from build123d import *

# Parameters (mm, degrees)
SKETCH1_W           = 400
SKETCH1_H           = 70
SKETCH1_R           = 30
SKETCH1_R_2         = 1.5
BOSS_EXTRUDE1_DEPTH = 3


with BuildPart() as part:
    # Sketch1 → Boss-Extrude1 (new body)
    with BuildSketch(Plane(origin=(0, 0, 0), x_dir=(1, 0, 0), z_dir=(0, 1, 0))):
        with Locations((200, 35)):
            Rectangle(SKETCH1_W, SKETCH1_H)
        with Locations(Location((40, 35, 0), (0, 0, 270))):
            Circle(SKETCH1_R, mode=Mode.SUBTRACT)
        with Locations(Location((120, 35, 0), (0, 0, 270))):
            Circle(SKETCH1_R, mode=Mode.SUBTRACT)
        with Locations(Location((200, 35, 0), (0, 0, 270))):
            Circle(SKETCH1_R, mode=Mode.SUBTRACT)
        with Locations(Location((280, 35, 0), (0, 0, 270))):
            Circle(SKETCH1_R, mode=Mode.SUBTRACT)
        with Locations(Location((360, 35, 0), (0, 0, 270))):
            Circle(SKETCH1_R, mode=Mode.SUBTRACT)
        with Locations(Location((15, 60, 0), (0, 0, 270))):
            Circle(SKETCH1_R_2, mode=Mode.SUBTRACT)
        with Locations(Location((65, 60, 0), (0, 0, 270))):
            Circle(SKETCH1_R_2, mode=Mode.SUBTRACT)
        with Locations(Location((65, 10, 0), (0, 0, 270))):
            Circle(SKETCH1_R_2, mode=Mode.SUBTRACT)
        with Locations(Location((15, 10, 0), (0, 0, 270))):
            Circle(SKETCH1_R_2, mode=Mode.SUBTRACT)
        with Locations(Location((95, 60, 0), (0, 0, 270))):
            Circle(SKETCH1_R_2, mode=Mode.SUBTRACT)
        with Locations(Location((145, 60, 0), (0, 0, 270))):
            Circle(SKETCH1_R_2, mode=Mode.SUBTRACT)
        with Locations(Location((145, 10, 0), (0, 0, 270))):
            Circle(SKETCH1_R_2, mode=Mode.SUBTRACT)
        with Locations(Location((95, 10, 0), (0, 0, 270))):
            Circle(SKETCH1_R_2, mode=Mode.SUBTRACT)
        with Locations(Location((175, 60, 0), (0, 0, 270))):
            Circle(SKETCH1_R_2, mode=Mode.SUBTRACT)
        with Locations(Location((225, 60, 0), (0, 0, 270))):
            Circle(SKETCH1_R_2, mode=Mode.SUBTRACT)
        with Locations(Location((225, 10, 0), (0, 0, 270))):
            Circle(SKETCH1_R_2, mode=Mode.SUBTRACT)
        with Locations(Location((175, 10, 0), (0, 0, 270))):
            Circle(SKETCH1_R_2, mode=Mode.SUBTRACT)
        with Locations(Location((255, 60, 0), (0, 0, 270))):
            Circle(SKETCH1_R_2, mode=Mode.SUBTRACT)
        with Locations(Location((305, 60, 0), (0, 0, 270))):
            Circle(SKETCH1_R_2, mode=Mode.SUBTRACT)
        with Locations(Location((305, 10, 0), (0, 0, 270))):
            Circle(SKETCH1_R_2, mode=Mode.SUBTRACT)
        with Locations(Location((255, 10, 0), (0, 0, 270))):
            Circle(SKETCH1_R_2, mode=Mode.SUBTRACT)
        with Locations(Location((335, 60, 0), (0, 0, 270))):
            Circle(SKETCH1_R_2, mode=Mode.SUBTRACT)
        with Locations(Location((385, 60, 0), (0, 0, 270))):
            Circle(SKETCH1_R_2, mode=Mode.SUBTRACT)
        with Locations(Location((385, 10, 0), (0, 0, 270))):
            Circle(SKETCH1_R_2, mode=Mode.SUBTRACT)
        with Locations(Location((335, 10, 0), (0, 0, 270))):
            Circle(SKETCH1_R_2, mode=Mode.SUBTRACT)
    extrude(amount=BOSS_EXTRUDE1_DEPTH)


solid = part.part
The model under review builds one solid part; all positions refer to its coordinate system, in mm. Coordinates: 2 decimals unless noted, no trailing zeros. Loops run counter-clockwise (first coordinate to the right, second up) from the corner with the lowest first, then second, coordinate; pieces in that order, holes last.
(1) Insertion check: P1, Ø2.5, axis at x = 385, z = -60, coming from the +Y side; P2, Ø5, axis at x = 95, z = -10, coming from the +Y side. Each pin has a flat end and moves straight along its axis. Give the tip position at first contact, or say it passes through.
Determined:
P1: passes through
P2: stops at y = 3
(2) Consider section A-A, the plane x = 280. Give the boundary of the cut face in (y, z).
Determined:
outline: (0, -70) - (3, -70) - (3, -65) - (0, -65) - close; (0, -5) - (3, -5) - (3, 0) - (0, 0) - close
(3) Consider section B-B, the plane z = -53. Give the boundary of the cut face in (x, y), plus the area to 3 significant figures.
Determined:
outline: (0, 0) - (16, 0) - (16, 3) - (0, 3) - close; (64, 0) - (96, 0) - (96, 3) - (64, 3) - close; (144, 0) - (176, 0) - (176, 3) - (144, 3) - close; (224, 0) - (256, 0) - (256, 3) - (224, 3) - close; (304, 0) - (336, 0) - (336, 3) - (304, 3) - close; (384, 0) - (400, 0) - (400, 3) - (384, 3) - close
area: 480 mm2
(4) Draft analysis for pull direction Z (two halves, no side actions). For faces 1 (the cylindrical face through (10.713, 1.479, -41.503)), 2 (the flat face through (197, 3, -4)), state which applies: +Z half, -Z half, draft (parallel to the pull), parting line (faces both ways), or undercut.
Determined:
face 1: undercut
face 2: draft
(5) Consider section C-C, the plane y = 1.7. Give the number of separate pieces and of enclosed holes in the cut face, plus the area to 3 significant figures.
Determined:
separate pieces: 1
enclosed holes: 25
area: 13,700 mm2
(6) Consider section D-D, the plane x = 196.5. Give the boundary of the cut face in (y, z), plus the area to 3 significant figures.
Determined:
outline: (0, -70) - (3, -70) - (3, -64.8) - (0, -64.8) - close; (0, -5.2) - (3, -5.2) - (3, 0) - (0, 0) - close
area: 31.2 mm2
(7) Wall thickness on L1, parallel to X at y = 2.25, z = -33; L2, parallel to Z at x = 65, y = 1.2; L3, parallel to Z at x = 281.5, y = 1.3: over which ranges is each line inside the solid? List them lowest first.
Determined:
L1: x = 0 to 10.07, 69.93 to 90.07, 149.93 to 170.07, 229.93 to 250.07, 309.93 to 330.07, 389.93 to 400
L2: z = -70 to -61.5, -58.5 to -51.58, -18.42 to -11.5, -8.5 to 0
L3: z = -70 to -64.96, -5.04 to 0
